Autodesk Inventor part; units mm, degrees
ref_plane "Work Plane1" through (75.5, 0, 0) normal (1, 0, 0) x (0, 0, -1)
ref_plane "YZ Plane" through (0, 0, 0) normal (1, 0, 0) x (0, 1, 0)
ref_plane "XZ Plane" through (0, 0, 0) normal (0, 1, 0) x (-1, 0, 0)
sketch "Sketch1" plane through (0, 0, 0) normal (1, 0, 0) x (0, 1, 0)
  line L0 (0, 0) -> (11, 0)
  line L1 (11, 0) -> (21.6853, -54.9711)
  line L2 (11, 0) -> (67, 0) construction
  line L3 (21.6853, -54.9711) -> (0, -59.1863)
  line L4 (21.6853, -54.9711) -> (43.7765, -54.9711) construction
  line L5 (0, -59.1863) -> (0, 0)
  dimension "d0" = 11
  dimension "d1" = 56
  dimension "d2" = 79
  dimension "d5" = 169
extrude "Extrusion1" add sketch "Sketch1" along normal blind 151
fillet "Fillet1" radius 2 4 edges at (151, 10.8427, -57.0787) (151, 5.5, 0) (0, 10.8427, -57.0787) (0, 5.5, 0)
sketch "Sketch2" plane through (2, 11, 0) normal (0, 0.9816, 0.1908) x (1, 0, 0)
  ellipse E0 centre (0, 2.0374) end of major axis (0, 0) minor radius 2 (-2, 2.0374) -> (0, 0) ccw
  line L0 (0, 0) -> (147, 0)
  ellipse E1 centre (147, 2.0374) end of major axis (147, 0) minor radius 2 (147, 0) -> (149, 2.0374) ccw
  line L1 (149, 54) -> (149, 2.0374)
  arc A0 (149, 54) -> (147, 56) centre (147, 54) ccw
  line L2 (0, 56) -> (147, 56)
  arc A1 (0, 56) -> (-2, 54) centre (0, 54) ccw
  line L3 (-2, 54) -> (-2, 2.0374)
  line L4 (2, 54) -> (145, 54)
  line L5 (147, 52) -> (147, 4)
  line L6 (145, 2) -> (2, 2)
  line L7 (0, 4) -> (0, 52)
  arc A2 (2, 54) -> (0, 52) centre (2, 52) ccw
  arc A3 (0, 4) -> (2, 2) centre (2, 4) ccw
  arc A4 (145, 2) -> (147, 4) centre (145, 4) ccw
  arc A5 (147, 52) -> (145, 54) centre (145, 52) ccw
  point P0 (-2, -2.0989)
  dimension "d7" = 2
  dimension "d8" = 2
  dimension "d9" = 2
  dimension "d10" = 2
  dimension "d11" = 2
extrude "Extrusion2" cut sketch "Sketch2" against normal blind 7 contours L4 A5 L5 A4 L6 A3 L7 A2
sketch "Sketch3" plane through (2, 4.1286, -1.3357) normal (0, 0.9816, 0.1908) x (1, 0, 0)
  line L0 (4, 52) -> (143, 52)
  line L1 (145, 50) -> (145, 6)
  line L2 (143, 4) -> (4, 4)
  line L3 (2, 6) -> (2, 50)
  line L4 (2, 54) -> (145, 54)
  line L5 (147, 52) -> (147, 4)
  line L6 (145, 2) -> (2, 2)
  line L7 (0, 4) -> (0, 52)
  arc A0 (4, 52) -> (2, 50) centre (4, 50) ccw
  arc A1 (2, 6) -> (4, 4) centre (4, 6) ccw
  arc A2 (143, 4) -> (145, 6) centre (143, 6) ccw
  arc A3 (145, 50) -> (143, 52) centre (143, 50) ccw
  point P0 (-2, -2.0989)
  dimension "d14" = 2
  dimension "d15" = 2
  dimension "d16" = 2
  dimension "d17" = 2
  dimension "d18" = 2
extrude "Extrusion3" cut sketch "Sketch3" against normal blind 3
ref_plane "Work Plane1" through (75.5, 0, 0) normal (1, 0, 0) x (0, 0, -1)
sketch "Sketch4" plane through (75.5, 0, 0) normal (1, 0, 0) x (0, 0, -1)
  line L0 (5.2622, 4.8918) -> (5.8346, 1.947)
  line L1 (50.9894, 10.7242) -> (7.7979, 2.3286)
  line L2 (52.3803, 14.0507) -> (52.9527, 11.1058)
  line L3 (5.8346, 1.947) -> (52.9527, 11.1058)
  line L4 (5.8346, 1.947) -> (7.7979, 2.3286)
  line L5 (5.8346, 1.947) -> (52.9527, 1.947)
  line L6 (52.9527, 1.947) -> (52.9527, 11.1058)
  line L7 (5.8346, 1.947) -> (52.9527, 11.1058)
  point P0 (0, 0)
  point P1 (7.7979, 2.3286)
extrude "Extrusion4" cut sketch "Sketch4" along normal mid plane 143
sketch "Sketch5" plane through (4, 1.947, -52.9527) normal (0, 0, 1) x (1, 0, 0)
  line L0 (0, 9.1588) -> (2, 9.1588)
  line L1 (0, 9.1588) -> (0, 0)
  line L2 (143, 0) -> (0, 0)
  line L3 (143, 0) -> (143, 9.1588)
  line L4 (141, 9.1588) -> (143, 9.1588)
  line L5 (2, 9.1588) -> (141, 9.1588)
  line L6 (66.75, 3.5) -> (76.25, 3.5)
  line L7 (76.25, 3.5) -> (76.25, 0)
  line L8 (76.25, 0) -> (66.75, 0)
  line L9 (66.75, 0) -> (66.75, 3.5)
  point P0 (-4, -1.947)
  point P1 (0, 4.5794)
  point P2 (71.5, 3.5)
  point P3 (76.25, 0)
  dimension "d24" = 9.5
  dimension "d25" = 3.5
  dimension "d26" = 0
  dimension "d27" = 71.5
  dimension "d28" = 71.5
extrude "Extrusion5" cut sketch "Sketch5" against normal blind 10 contours L9 L6 L7 L2
properties part number "housing"
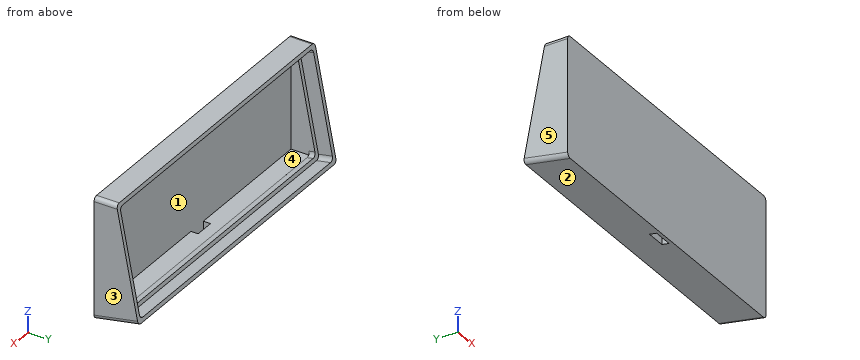
Work out the finished part from the listing and answer in its coordinate system (mm). Face numbers are marked on the shaded views. A direction names the side the tool comes from. Coordinates: 2 decimals unless noted, no trailing zeros. Write each loop counter-clockwise with the first axis right and the second up, starting at its lowest first coordinate (ties: lowest second). Pieces come first, ordered by that corner, then holes. Notation, with made-up numbers: (0.25, -22) - (28.25, -22) arc R23 cw to (28.25, 10) - close; hole circle Ø5 at (-4.5, -27.75). An arc over 180 degrees is marked (long way). Answer as a JSON object with one key per item and string values.
Q1. Find section B-B (z = -16). Write down the section's boundary in (x, y), plus the area to 3 significant figures.
Results list:
{"outline": "(0, 0) - (151, 0) - (151, 14.11) - (149, 14.11) - (149, 6.98) - (147, 6.98) - (147, 1.95) - (4, 1.95) - (4, 6.98) - (2, 6.98) - (2, 14.11) - (0, 14.11) - close", "area": "363 mm^2"}
Q2. Consider L1, parallel to X at y = 13, z = -18; L2, parallel to X at y = 3, z = -30; L3, parallel to Y at x = 64, z = -12. Determine where each line is inside the solid, lowest interval first. Write a range as from..to.
Results list:
{"L1": "x = 0..2, 149..151", "L2": "x = 0..4, 147..151", "L3": "y = 0..1.95"}
Q3. Which of the six approach directions +Z, -Z, +X, -X, +Y, -Y give full straight-line access (tool end or side, diameter ignored) to the marked faces 4 and 5?
Results list:
{"face 4": "none", "face 5": "+Z, -Z, -X, +Y, -Y"}
Q4. For a pull along Z with two mould halves and no side action, classify the marked faces 1, 2 and 3 as pulls with the +Z half, pulls with the -Z half, needs draft (parallel to the pull), parting line crosses it, or undercut.
Results list:
{"face 1": "undercut", "face 2": "pulls with the -Z half", "face 3": "needs draft"}
Q5. Find section C-C (z = -35). Write down the section's boundary in (x, y).
Results list:
{"outline": "(0, 0) - (151, 0) - (151, 17.8) - (149, 17.8) - (149, 10.67) - (147, 10.67) - (147, 1.95) - (4, 1.95) - (4, 10.67) - (2, 10.67) - (2, 17.8) - (0, 17.8) - close"}
Q6. Given pin 1 Ø10 at (x, z) = (44.5, -45) entering from +Y, flat-ended and moving along its own axis, determine where the tip first touches the part or whether it passes through.
Results list:
{"pin 1": "stops at y = 1.95"}
